```python
from build123d import *

# Parameters (mm, degrees)
SKETCH1_W            = 198
SKETCH1_H            = 108
BOSS_EXTRUDE1_DEPTH  = 40
SKETCH4_W            = 181
SKETCH4_H            = 45
CUT_EXTRUDE2_DEPTH   = 10
CUT_EXTRUDE3_DEPTH   = 175
BOSS_EXTRUDE11_DEPTH = 10
CUT_EXTRUDE12_DEPTH  = 175
CUT_EXTRUDE28_DEPTH  = 14.5
CUT_EXTRUDE29_DEPTH  = 14.5
CUT_EXTRUDE40_REACH  = 231.059
CUT_EXTRUDE5_DEPTH   = 23
SKETCH12_R           = 3.15
CUT_EXTRUDE9_DEPTH   = 230.058944379
SKETCH13_R           = 4.5
CUT_EXTRUDE10_DEPTH  = 16.5
SKETCH14_R           = 4.5
CUT_EXTRUDE11_DEPTH  = 16.5
SKETCH41_R           = 2.9
CUT_EXTRUDE21_DEPTH  = 7
CUT_EXTRUDE22_DEPTH  = 10
CUT_EXTRUDE23_DEPTH  = 10
SKETCH6_W            = 141.2
SKETCH6_H            = 21.2
CUT_EXTRUDE32_DEPTH  = 2.3
SKETCH23_W           = 141.2
SKETCH23_H           = 21.2
CUT_EXTRUDE33_DEPTH  = 2.3
CUT_EXTRUDE34_DEPTH  = 55.4
CUT_EXTRUDE35_DEPTH  = 55.4
CUT_EXTRUDE36_DEPTH  = 55.4
SKETCH90_R           = 6.1
CUT_EXTRUDE38_DEPTH  = 17
SKETCH96_R           = 2
CUT_EXTRUDE39_DEPTH  = 230.058944379
SKETCH98_R           = 7.5
CUT_EXTRUDE41_DEPTH  = 4


with BuildPart() as part:
    # Sketch1 → Boss-Extrude1 (new body)
    with BuildSketch(Plane(origin=(0, 0, 0), x_dir=(1, 0, 0), z_dir=(0, 1, 0))):
        with Locations((99, 54)):
            Rectangle(SKETCH1_W, SKETCH1_H)
    extrude(amount=BOSS_EXTRUDE1_DEPTH)

    # Sketch4 → Cut-Extrude2 (cut)
    with BuildSketch(Plane(origin=(0, 0, 0), x_dir=(1, 0, 0), z_dir=(0, 1, 0))):
        with Locations((99, 54)):
            Rectangle(SKETCH4_W, SKETCH4_H)
    extrude(amount=CUT_EXTRUDE2_DEPTH, mode=Mode.SUBTRACT)

    # Sketch5 → Cut-Extrude3 (cut)
    with BuildSketch(Plane(origin=(198, 0, 0), x_dir=(0, 0, -1), z_dir=(1, 0, 0))):
        Polygon((54, 40), (108, 33.828382143), (108, 40), align=None)
    extrude(amount=-CUT_EXTRUDE3_DEPTH, mode=Mode.SUBTRACT)

    # Sketch53 → Boss-Extrude11 (add)
    with BuildSketch(Plane(origin=(0, 10, 0), x_dir=(-1, 0, 0), z_dir=(0, -1, 0))):
        Polygon((-8.5, 51.5), (-8.5, 31.5), (-39.5, 31.5), align=None)
        Polygon((-8.5, 56.5), (-8.5, 76.5), (-39.5, 76.5), align=None)
        Polygon((-158.5, 76.5), (-189.5, 56.5), (-189.5, 76.5), align=None)
        Polygon((-158.5, 31.5), (-189.5, 51.5), (-189.5, 31.5), align=None)
    extrude(amount=BOSS_EXTRUDE11_DEPTH)

    # Sketch18 → Cut-Extrude12 (cut)
    with BuildSketch(Plane(origin=(198, 0, 0), x_dir=(0, 0, -1), z_dir=(1, 0, 0))):
        Polygon((0, 33.828382143), (0, 40), (54, 40), align=None)
    extrude(amount=-CUT_EXTRUDE12_DEPTH, mode=Mode.SUBTRACT)

    # Izq → Cut-Extrude28 (cut)
    with BuildSketch(Plane(origin=(0, 28.012686094, -12.204810084), x_dir=(1, 0, 0), z_dir=(0, 0.9167660546215652, -0.39942458749256926))):
        Polygon((8.5, 48.862182113), (29.5, 70.132603179), (8.5, 70.132603179), align=None)
    cut_extrude28 = extrude(amount=-CUT_EXTRUDE28_DEPTH, mode=Mode.SUBTRACT)

    # Der → Cut-Extrude29 (cut)
    with BuildSketch(Plane(origin=(0, -11.144923858, -4.62106599), x_dir=(1, 0, 0), z_dir=(0, 0.9237421135716327, 0.38301502270043264))):
        Polygon((8.5, 51.290217599), (29.5, 29.097876578), (8.5, 29.097876578), align=None)
    cut_extrude29 = extrude(amount=-CUT_EXTRUDE29_DEPTH, mode=Mode.SUBTRACT)

    # Cut-Extrude40: up to this face of the body (flat: up to its plane)
    cut_extrude40_end = Plane(part.part.faces().sort_by_distance((99, 10, -54))[0])
    # Sketch97 → Cut-Extrude40 (cut, up to the picked face)
    with BuildSketch(Plane(origin=(0, 0, 0), x_dir=(1, 0, 0), z_dir=(0, 1, 0)), mode=Mode.PRIVATE) as cut_extrude40_sk1:
        Polygon((8.5, 57.5), (29.5, 76.5), (158.5, 76.5), (189.5, 56.5), (189.5, 51.5), (158.5, 31.5), (29.5, 31.5), (8.5, 51.5), align=None)
    cut_extrude40_tool1 = split(extrude(cut_extrude40_sk1.sketch, amount=CUT_EXTRUDE40_REACH, mode=Mode.PRIVATE), bisect_by=cut_extrude40_end, keep=Keep.BOTH, mode=Mode.PRIVATE)
    cut_extrude40 = cut_extrude40_tool1.solids().sort_by(Axis((96.82024, 0, -54.014019), (0, 1, 0)))[0]
    add(cut_extrude40, mode=Mode.SUBTRACT)

    # Mirror2: Cut-Extrude28, Cut-Extrude29, Cut-Extrude40 across plane
    add(cut_extrude28.mirror(Plane(origin=(99, 0, 0), x_dir=(0, 0, 1), z_dir=(1, 0, 0))), mode=Mode.SUBTRACT)
    add(cut_extrude29.mirror(Plane(origin=(99, 0, 0), x_dir=(0, 0, 1), z_dir=(1, 0, 0))), mode=Mode.SUBTRACT)
    add(cut_extrude40.mirror(Plane(origin=(99, 0, 0), x_dir=(0, 0, 1), z_dir=(1, 0, 0))), mode=Mode.SUBTRACT)

    # Sketch7 → Cut-Extrude5 (cut)
    with BuildSketch(Plane(origin=(0, 0, 0), x_dir=(0, 0, -1), z_dir=(1, 0, 0))):
        Polygon((108, 40), (108, 35), (83.505102572, 40), align=None)
        Polygon((0, 35), (0, 40), (24.494897428, 40), align=None)
    extrude(amount=CUT_EXTRUDE5_DEPTH, mode=Mode.SUBTRACT)

    # Sketch12 → Cut-Extrude9 (cut, through all)
    with BuildSketch(Plane(origin=(0, 40, 0), x_dir=(1, 0, 0), z_dir=(0, 1, 0))):
        with Locations(Location((19.7, 98.85, 0), (0, 0, 270))):
            Circle(SKETCH12_R)
        with Locations(Location((99.7, 9.15, 0), (0, 0, 270))):
            Circle(SKETCH12_R)
        with Locations(Location((179.7, 9.15, 0), (0, 0, 270))):
            Circle(SKETCH12_R)
        with Locations(Location((19.7, 9.15, 0), (0, 0, 270))):
            Circle(SKETCH12_R)
        with Locations(Location((99.7, 98.85, 0), (0, 0, 270))):
            Circle(SKETCH12_R)
        with Locations(Location((179.7, 98.85, 0), (0, 0, 270))):
            Circle(SKETCH12_R)
    extrude(amount=-CUT_EXTRUDE9_DEPTH, mode=Mode.SUBTRACT)

    # Sketch13 → Cut-Extrude10 (cut)
    with BuildSketch(Plane(origin=(0, 45.576299066, -5.208879651), x_dir=(1, 0, 0), z_dir=(0, 0.9935322797694506, -0.11355002886885623))):
        with Locations(Location((46.5, 90.460272446, 0), (0, 0, 270))):
            Circle(SKETCH13_R)
        with Locations(Location((151.5, 90.460272446, 0), (0, 0, 270))):
            Circle(SKETCH13_R)
    extrude(amount=-CUT_EXTRUDE10_DEPTH, mode=Mode.SUBTRACT)

    # Sketch14 → Cut-Extrude11 (cut)
    with BuildSketch(Plane(origin=(0, 33.058773264, 6.733871157), x_dir=(1, 0, 0), z_dir=(0, 0.9935322797694507, 0.11355002886885664))):
        with Locations(Location((46.5, 19.910744715, 0), (0, 0, 270))):
            Circle(SKETCH14_R)
        with Locations(Location((151.5, 19.910744715, 0), (0, 0, 270))):
            Circle(SKETCH14_R)
    extrude(amount=-CUT_EXTRUDE11_DEPTH, mode=Mode.SUBTRACT)

    # Sketch41 → Cut-Extrude21 (cut)
    with BuildSketch(Plane(origin=(0, 0, 0), x_dir=(1, 0, 0), z_dir=(0, 1, 0))):
        with Locations(Location((139.5, 9, 0), (0, 0, 90))):
            Circle(SKETCH41_R)
        with Locations(Location((139.5, 99, 0), (0, 0, 90))):
            Circle(SKETCH41_R)
    extrude(amount=CUT_EXTRUDE21_DEPTH, mode=Mode.SUBTRACT)

    # Sketch42 → Cut-Extrude22 (cut)
    with BuildSketch(Plane.XY):
        with BuildLine():
            Line((142.3, 12.8), (152, 12.8))
            ThreePointArc((152, 12.8), (153.8, 11), (152, 9.2))
            Line((152, 9.2), (142.3, 9.2))
            ThreePointArc((142.3, 9.2), (140.5, 11), (142.3, 12.8))
        make_face()
    extrude(amount=-CUT_EXTRUDE22_DEPTH, mode=Mode.SUBTRACT)

    # Sketch43 → Cut-Extrude23 (cut)
    with BuildSketch(Plane(origin=(0, 0, -108), x_dir=(-1, 0, 0), z_dir=(0, 0, -1))):
        with BuildLine():
            Line((-55.7, 12.8), (-46, 12.8))
            ThreePointArc((-46, 12.8), (-44.2, 11), (-46, 9.2))
            Line((-46, 9.2), (-55.7, 9.2))
            ThreePointArc((-55.7, 9.2), (-57.5, 11), (-55.7, 12.8))
        make_face()
    extrude(amount=-CUT_EXTRUDE23_DEPTH, mode=Mode.SUBTRACT)

    # Sketch6 → Cut-Extrude32 (cut)
    with BuildSketch(Plane(origin=(0, 45.576299066, -5.208879651), x_dir=(1, 0, 0), z_dir=(0, 0.9935322797694506, -0.11355002886885623))):
        with BuildLine():
            Line((28.9, 76.508741953), (169.5, 76.508741953))
            ThreePointArc((169.5, 76.508741953), (171.621320344, 75.630062296), (172.5, 73.508741953))
            Line((172.5, 73.508741953), (172.5, 52.908741953))
            ThreePointArc((172.5, 52.908741953), (171.621320344, 50.787421609), (169.5, 49.908741953))
            Line((169.5, 49.908741953), (28.9, 49.908741953))
            ThreePointArc((28.9, 49.908741953), (26.778679656, 50.787421609), (25.9, 52.908741953))
            Line((25.9, 52.908741953), (25.9, 73.508741953))
            ThreePointArc((25.9, 73.508741953), (26.778679656, 75.630062296), (28.9, 76.508741953))
        make_face()
        with Locations((99.2, 63.208741953)):
            Rectangle(SKETCH6_W, SKETCH6_H, mode=Mode.SUBTRACT)
    extrude(amount=-CUT_EXTRUDE32_DEPTH, mode=Mode.SUBTRACT)

    # Sketch23 → Cut-Extrude33 (cut)
    with BuildSketch(Plane(origin=(0, 33.392212209, 3.816369873), x_dir=(1, 0, 0), z_dir=(0, 0.9935322797694506, 0.11355002886885662))):
        with BuildLine():
            Line((28.9, 57.392744262), (169.5, 57.392744262))
            ThreePointArc((169.5, 57.392744262), (171.621320344, 56.514064606), (172.5, 54.392744262))
            Line((172.5, 54.392744262), (172.5, 33.792744262))
            ThreePointArc((172.5, 33.792744262), (171.621320344, 31.671423919), (169.5, 30.792744262))
            Line((169.5, 30.792744262), (28.9, 30.792744262))
            ThreePointArc((28.9, 30.792744262), (26.778679656, 31.671423919), (25.9, 33.792744262))
            Line((25.9, 33.792744262), (25.9, 54.392744262))
            ThreePointArc((25.9, 54.392744262), (26.778679656, 56.514064606), (28.9, 57.392744262))
        make_face()
        with Locations((99.2, 44.092744262)):
            Rectangle(SKETCH23_W, SKETCH23_H, mode=Mode.SUBTRACT)
    extrude(amount=-CUT_EXTRUDE33_DEPTH, mode=Mode.SUBTRACT)

    # Sketch83 → Cut-Extrude34 (cut)
    with BuildSketch(Plane(origin=(0, 33.392212209, 3.816369873), x_dir=(1, 0, 0), z_dir=(0, 0.9935322797694506, 0.11355002886885662))):
        with BuildLine():
            Line((31.7, 54.092744262), (166.7, 54.092744262))
            ThreePointArc((166.7, 54.092744262), (168.467766953, 53.360511215), (169.2, 51.592744262))
            Line((169.2, 51.592744262), (169.2, 36.592744262))
            ThreePointArc((169.2, 36.592744262), (168.467766953, 34.824977309), (166.7, 34.092744262))
            Line((166.7, 34.092744262), (31.7, 34.092744262))
            ThreePointArc((31.7, 34.092744262), (29.932233047, 34.824977309), (29.2, 36.592744262))
            Line((29.2, 36.592744262), (29.2, 51.592744262))
            ThreePointArc((29.2, 51.592744262), (29.932233047, 53.360511215), (31.7, 54.092744262))
        make_face()
    extrude(amount=-CUT_EXTRUDE34_DEPTH, mode=Mode.SUBTRACT)

    # Sketch84 → Cut-Extrude35 (cut)
    with BuildSketch(Plane(origin=(0, 45.576299066, -5.208879651), x_dir=(1, 0, 0), z_dir=(0, 0.9935322797694506, -0.11355002886885623))):
        with BuildLine():
            Line((31.7, 53.208741953), (166.7, 53.208741953))
            ThreePointArc((166.7, 53.208741953), (168.467766953, 53.940975), (169.2, 55.708741953))
            Line((169.2, 55.708741953), (169.2, 70.708741953))
            ThreePointArc((169.2, 70.708741953), (168.467766953, 72.476508906), (166.7, 73.208741953))
            Line((166.7, 73.208741953), (31.7, 73.208741953))
            ThreePointArc((31.7, 73.208741953), (29.932233047, 72.476508906), (29.2, 70.708741953))
            Line((29.2, 70.708741953), (29.2, 55.708741953))
            ThreePointArc((29.2, 55.708741953), (29.932233047, 53.940975), (31.7, 53.208741953))
        make_face()
    extrude(amount=-CUT_EXTRUDE35_DEPTH, mode=Mode.SUBTRACT)

    # Sketch85 → Cut-Extrude36 (cut)
    with BuildSketch(Plane(origin=(0, 40, 0), x_dir=(1, 0, 0), z_dir=(0, 1, 0))):
        Polygon((0, 101.9), (6.1, 108), (0, 108), align=None)
        Polygon((0, 0), (6.1, 0), (0, 6.1), align=None)
        Polygon((198, 6.1), (191.9, 0), (198, 0), align=None)
        Polygon((198, 108), (191.9, 108), (198, 101.9), align=None)
    extrude(amount=-CUT_EXTRUDE36_DEPTH, mode=Mode.SUBTRACT)

    # Sketch90 → Cut-Extrude38 (cut)
    with BuildSketch(Plane(origin=(0, 40, 0), x_dir=(1, 0, 0), z_dir=(0, 1, 0))):
        with Locations(Location((19.7, 9.15, 0), (0, 0, 270))):
            Circle(SKETCH90_R)
        with Locations(Location((99.7, 9.15, 0), (0, 0, 270))):
            Circle(SKETCH90_R)
        with Locations(Location((179.7, 9.15, 0), (0, 0, 270))):
            Circle(SKETCH90_R)
        with Locations(Location((99.7, 98.85, 0), (0, 0, 270))):
            Circle(SKETCH90_R)
        with Locations(Location((179.7, 98.85, 0), (0, 0, 270))):
            Circle(SKETCH90_R)
        with Locations(Location((19.7, 98.85, 0), (0, 0, 270))):
            Circle(SKETCH90_R)
    extrude(amount=-CUT_EXTRUDE38_DEPTH, mode=Mode.SUBTRACT)

    # Sketch96 → Cut-Extrude39 (cut, through all)
    with BuildSketch(Plane(origin=(0, 0, 0), x_dir=(1, 0, 0), z_dir=(0, 1, 0))):
        with Locations(Location((15.45, 54, 0), (0, 0, 270))):
            Circle(SKETCH96_R)
        with Locations((185, 54)):
            Circle(SKETCH96_R)
    extrude(amount=CUT_EXTRUDE39_DEPTH, mode=Mode.SUBTRACT)

    # Sketch98 → Cut-Extrude41 (cut)
    with BuildSketch(Plane(origin=(0, 40, 0), x_dir=(1, 0, 0), z_dir=(0, 1, 0))):
        with Locations(Location((185, 54, 0), (0, 0, 270))):
            Circle(SKETCH98_R)
    extrude(amount=-CUT_EXTRUDE41_DEPTH, mode=Mode.SUBTRACT)


solid = part.part
```
Source: CAD feature listing. Evaluate the final solid. Frame: model axes, mm. A direction names the side the tool comes from. Give positions to 0.01 mm unless a question says otherwise; leave off trailing zeros. Order: outer loops, then holes, each group sorted by start corner. A loop starts at its lowest first (then second) coordinate and runs counter-clockwise, first axis right, second up.
(1) Access query for faces 5 (the face through (23, 38, -30)), 6 (the face through (142.33, 3.45, -98.37)), 7 (the face through (110.4, 34.89, -29.55)), 8 (the face through (179.968, 29.407, -15.244)), 9 (the face through (23, 38, -78)). Directions: +Z, -Z, +X, -X, +Y, -Y. A direction counts if a zero-diameter tool reaches every point of the face in a straight line with its end or side. Return the directions, or none.
(2) Contact query for flat-ended pins moving along their axis: P1, Ø6, axis at x = 29.5, z = -59.5, coming from the -Y side; P2, Ø1.7, axis at x = 138.5, z = -8.5, coming from the -Y side; P3, Ø5, axis at x = 145.5, z = -4.5, coming from the +Y side. Output: stop coordinate, or through.
(3) Pull-direction query (Y, two-part tool) for faces 1 (the face through (153.8, 11, -4.9)), 2 (the face through (29.95, 23.76, -32.32)), 3 (the face through (25.9, 37, -40)), 4 (the face through (147.107, 27.349, -14.941)); classes: +Y half, -Y half, draft (parallel to the pull), parting line (faces both ways), or undercut.
(4) Section query C-C (x = 19.7). Return the cut outline in (y, z).
(5) Section query A-A (x = 127.5). State how many separate pieces and enclosed holes the cut face has, plus the area to 3 significant figures.
(6) Material intervals for line 1 along X through (y, z) = (16, -98.85); line 2 along Z through (x, y) = (179, 28); line 3 along X through (y, z) = (25, -99), sorted ascending.
Outcome:
1. face 5: +Z, +X, +Y
1. face 6: -Y
1. face 7: none
1. face 8: +Y
1. face 9: -Z, +X, +Y
2. P1: stops at y = 10
2. P2: stops at y = 7
2. P3: stops at y = 34.63
3. face 1: undercut
3. face 2: +Y half
3. face 3: draft
3. face 4: undercut
4. outline: (0, -108) - (35, -108) - (35.62, -104.95) - (23, -104.95) - (23, -102) - (0, -102) - close; (0, -95.7) - (23, -95.7) - (23, -92.75) - (38.11, -92.75) - (40, -83.51) - (40, -24.49) - (38.11, -15.25) - (23, -15.25) - (23, -12.3) - (0, -12.3) - (0, -31.5) - (3.87, -40.83) - (10, -40.83) - (10, -67.63) - (3.86, -67.63) - (0, -76.5) - close; (0, -6) - (23, -6) - (23, -3.05) - (35.62, -3.05) - (35, 0) - (0, 0) - close
5. separate pieces: 3
5. enclosed holes: 0
5. area: 2,370 mm2
6. line 1: x = 0 to 16.55, 22.85 to 96.55, 102.85 to 176.55, 182.85 to 198
6. line 2: z = -108 to -104.91, -92.79 to -15.21, -3.09 to 0
6. line 3: x = 0 to 13.6, 25.8 to 93.6, 105.8 to 173.6, 185.8 to 198
